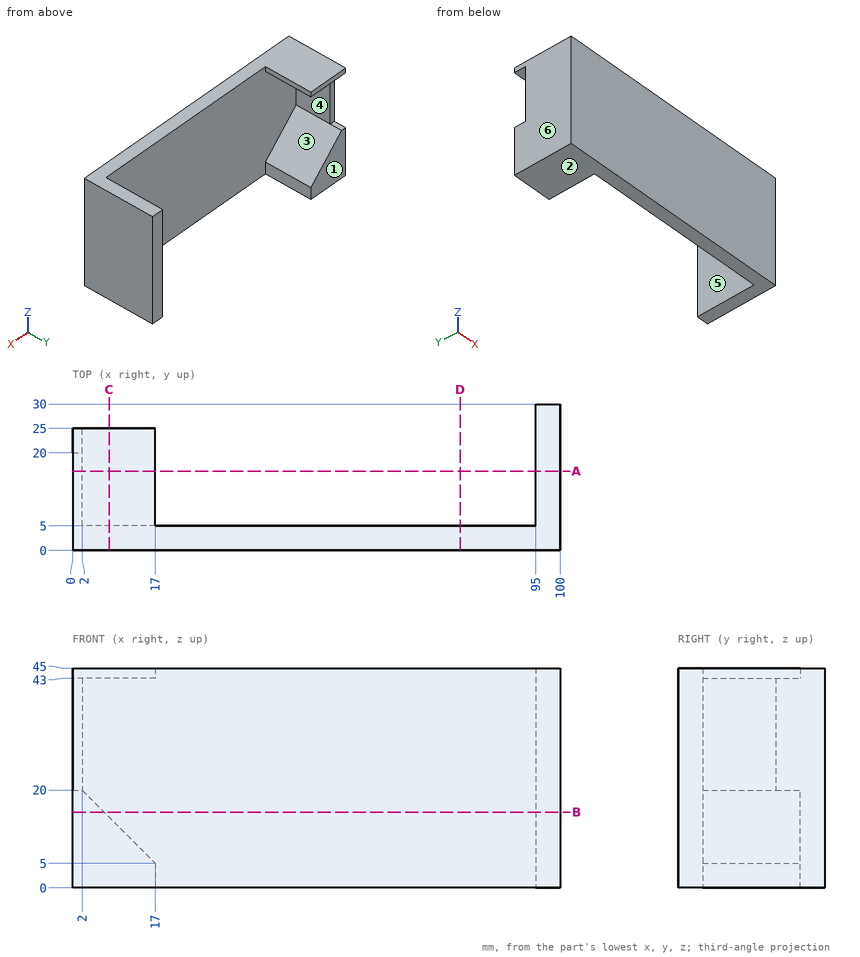
Geometry check sheet. Reference: drawing and pictorial views, mm from the part's lowest x, y, z. A direction names the side the tool comes from. Give positions to 0.01 mm unless a question says otherwise; leave off trailing zeros. Order: outer loops, then holes, each group sorted by start corner. A loop starts at its lowest first (then second) coordinate and runs counter-clockwise, first axis right, second up. Notation, with made-up numbers: (55.25, 18.25) - (82.25, 18.25) arc R27 ccw to (82.25, 50.25) - close; hole circle Ø2 at (-21.5, 39.5). An arc over 180 degrees is marked (long way). Answer as CSV lines item,"result".
1. Section check D-D (x = 79.5). Record the boundary of the cut face in (y, z), then the cut area to 3 significant figures.
Result sheet:
outline,"(0, 0) - (5, 0) - (5, 45) - (0, 45) - close"
area,"225 mm²"
2. Go/stop test with flat-tipped pins: P1, Ø3, axis at x = 78, z = 20.5, coming from the +Y side; P2, Ø1.6, axis at x = 5.5, z = 44, coming from the +Y side; P3, Ø1.6, axis at x = 1, z = 26.5, coming from the +Y side. Record where each tip stops, or that it passes through.
Result sheet:
P1,"y = 5"
P2,"y = 25"
P3,"y = 20"
3. Mould release check, pull along Z, two halves, no side actions. Record for the marked faces 1, 2, 3 and 4: released by +Z, released by -Z, zero draft, split by the parting line, or undercut.
Result sheet:
face 1,"zero draft"
face 2,"released by -Z"
face 3,"undercut"
face 4,"undercut"
4. Tool access check on the marked faces 5 and 6. Record the directions out of +Z, -Z, +X, -X, +Y, -Y that give a thin tool (end or side, any length) a straight path to the whole face; none if there is none.
Result sheet:
face 5,"+Z, -Z, +Y"
face 6,"+Z, -Z, -X, +Y, -Y"
5. Section check B-B (z = 15.5). Record the boundary of the cut face in (x, y).
Result sheet:
outline,"(0, 0) - (100, 0) - (100, 30) - (95, 30) - (95, 5) - (6.5, 5) - (6.5, 25) - (0, 25) - close"
6. Scan lines: probe 1 along X at (y, z) = (11, 25.5); probe 2 along Y at (x, z) = (8, 41); probe 3 along Y at (x, z) = (6, 6.5). Record each from-to range of solid material in increasing order. Write a range as from..to.
Result sheet:
probe 1,"0..2, 95..100"
probe 2,"0..5"
probe 3,"0..25"
7. Section check C-C (x = 7.5). Record the boundary of the cut face in (y, z).
Result sheet:
outline,"(0, 0) - (25, 0) - (25, 14.5) - (5, 14.5) - (5, 43) - (25, 43) - (25, 45) - (0, 45) - close"
8. Section check A-A (y = 16.25). Record the boundary of the cut face in (x, z), then the cut area to 4 significant figures.
Result sheet:
outline,"(0, 0) - (17, 0) - (17, 5) - (2, 20) - (2, 43) - (17, 43) - (17, 45) - (0, 45) - close; (95, 0) - (100, 0) - (100, 45) - (95, 45) - close"
area,"532.5 mm²"
